Work out the finished part from the listing and answer in its coordinate system (mm). A direction names the side the tool comes from. Give positions to 0.01 mm unless a question says otherwise; leave off trailing zeros. Loops run counter-clockwise (first coordinate to the right, second up) from the corner with the lowest first, then second, coordinate; pieces in that order, holes last. Notation, with made-up numbers: (-15, -25) -> (39, -25) arc R22 cw to (39, -4) -> close; hole circle Ø4 at (4, 6.5). An arc over 180 degrees is marked (long way). Answer as CSV lines item,"result". Start each with the question number.
1. Determine the mould class of faces 1 (the face through (-7.5, -1, 2)), 2 (the face through (0, 5, 1.8)), 3 (the face through (5, 2, 3)) for opening direction X: +X half, -X half, draft (parallel to the pull), parting line (faces both ways), or undercut.
2. Find section A-A, the plane x = -4.5. Give the vertices of the cut face in (y, z), and give its area (3 significant figures).
3. Find section C-C, the plane x = 3. Give the vertices of the cut face in (y, z), and give its area (4 significant figures).
4. Find the intervals of material crossed by line 1 along X through (y, z) = (1.4, 0); line 2 along Z through (x, y) = (1, 0.25); line 3 along X through (y, z) = (1, -1), in increasing order.
5. Find section B-B, the plane y = -0.5. Give the vertices of the cut face in (x, z).
6. Find section D-D, the plane z = 2.25. Give the vertices of the cut face in (x, y).
7. A tool of negligible diameter and unlimited length cuts with its end or side. For faces 4 (the face through (2, -1, 4)), 5 (the face through (-5, 3, 1)), 6 (the face through (4, -1, 6)), from which of +Z, -Z, +X, -X, +Y, -Y can it reach the whole face along a straight path? Write none if from no direction.
8. Flat-ended cylindrical pins translate along their axes: pin 1 Ø1.5 at (x, y) = (3.5, 4) entering from -Z; pin 2 Ø2.5 at (x, y) = (0, 5) entering from +Z; pin 3 Ø2 at (x, y) = (-4.5, 5.5) entering from -Z. Find the tip coordinate at first contact, or state that the pin passes through.
from build123d import *

# Parameters (mm, degrees)
SKETCH1_W           = 10
SKETCH1_H           = 10
BOSS_EXTRUDE1_DEPTH = 10
SKETCH2_R           = 1.6
CUT_EXTRUDE1_DEPTH  = 3.2
SKETCH3_R           = 1.6
CUT_EXTRUDE3_DEPTH  = 3.2
SKETCH4_R           = 1.6
CUT_EXTRUDE4_DEPTH  = 3.2
CHAMFER1_SIZE       = 6
BOSS_EXTRUDE2_DEPTH = 2.5


with BuildPart() as part:
    # Sketch1 → Boss-Extrude1 (new body)
    with BuildSketch(Plane(origin=(0, 0, 0), x_dir=(1, 0, 0), z_dir=(0, 1, 0))):
        Rectangle(SKETCH1_W, SKETCH1_H)
    extrude(amount=BOSS_EXTRUDE1_DEPTH)

    # Sketch2 → Cut-Extrude1 (cut)
    with BuildSketch(Plane.XY.offset(5)):
        with Locations((0, 5)):
            Circle(SKETCH2_R)
    extrude(amount=-CUT_EXTRUDE1_DEPTH, mode=Mode.SUBTRACT)

    # Sketch3 → Cut-Extrude3 (cut)
    with BuildSketch(Plane(origin=(0, 0, 0), x_dir=(-1, 0, 0), z_dir=(0, -1, 0))):
        with Locations(Location((0, 0, 0), (0, 0, 90))):
            Circle(SKETCH3_R)
    extrude(amount=-CUT_EXTRUDE3_DEPTH, mode=Mode.SUBTRACT)

    # Sketch4 → Cut-Extrude4 (cut)
    with BuildSketch(Plane(origin=(-5, 0, 0), x_dir=(0, 0, -1), z_dir=(1, 0, 0))):
        with Locations((0, 5)):
            Circle(SKETCH4_R)
    extrude(amount=CUT_EXTRUDE4_DEPTH, mode=Mode.SUBTRACT)

    # Chamfer1
    chamfer1_edges = [part.edges().sort_by_distance(p)[0] for p in [
        (5, 10, 0),
        (5, 5, -5),
        (0, 10, -5),
    ]]
    chamfer(chamfer1_edges, length=CHAMFER1_SIZE)

    # Sketch5 → Boss-Extrude2 (add)
    with BuildSketch(Plane(origin=(0, -2.5, 0), x_dir=(-1, 0, 0), z_dir=(0, -1, 0))):
        with BuildLine():
            Line((-4, -4), (-4, -7.5))
            Line((-4, -7.5), (7.5, -7.5))
            Line((7.5, -7.5), (7.5, 4))
            Line((7.5, 4), (4, 4))
            Line((4, 4), (4, 0))
            ThreePointArc((4, 0), (2.828427125, -2.828427125), (0, -4))
            Line((0, -4), (-4, -4))
        make_face()
    extrude(amount=-BOSS_EXTRUDE2_DEPTH)


solid = part.part
Resolved:
1,face 1,"-X half"
1,face 2,"undercut"
1,face 3,"+X half"
2,outline,"(-2.5, -4) -> (0, -4) -> (0, -5) -> (4, -5) -> (10, 1) -> (10, 5) -> (0, 5) -> (0, 7.5) -> (-2.5, 7.5) -> close; hole circle Ø3.2 at (5, 0)"
2,area,"103 mm^2"
3,outline,"(-2.5, 4) -> (0, 4) -> (0, -1) -> (4, -1) -> (6, 1) -> (6, 5) -> (0, 5) -> (0, 7.5) -> (-2.5, 7.5) -> close"
3,area,"42.75 mm^2"
4,line 1,"x = -5 to -1.6, 1.6 to 4"
4,line 2,"z = -3 to -1.25, 1.25 to 5"
4,line 3,"x = -5 to -1.25, 1.25 to 3"
5,outline,"(-7.5, -4) -> (-4, -4) -> (-4, 0) arc R4 cw to (0, 4) -> (4, 4) -> (4, 7.5) -> (-7.5, 7.5) -> close"
6,outline,"(-7.5, -2.5) -> (-3.31, -2.5) -> (-3.31, 0) -> (5, 0) -> (5, 4) -> (-1, 10) -> (-5, 10) -> (-5, 0) -> (-7.5, 0) -> close; hole circle Ø3.2 at (0, 5)"
7,face 4,"-Z, +X, -Y"
7,face 5,"+Z, -Z, -X, +Y"
7,face 6,"+Z, -Z, +X, -Y"
8,pin 1,"stops at z = -1.25"
8,pin 2,"stops at z = 1.8"
8,pin 3,"stops at z = -4.5"
